Here's how the part is built. I have some questions about the finished solid (model axes, mm). Coordinates: 2 decimals unless noted, no trailing zeros. Write each loop counter-clockwise with the first axis right and the second up, starting at its lowest first coordinate (ties: lowest second). Pieces come first, ordered by that corner, then holes. Notation, with made-up numbers: (52.5, 71) -> (100.5, 71) arc R18 cw to (100.5, 86) -> close; hole circle Ø9 at (88, 40.25). An arc over 180 degrees is marked (long way). Use a Markdown table: item, result. Add a question column.
Item 1: Imagine slicing it at D-D, the plane x = 1.05. Count the separate pieces of the cut face and the enclosed holes in it, and give its area (3 significant figures).
Item 2: Imagine slicing it at B-B, the plane y = 10.3. Write out the boundary of the cut face in (x, z), and give its area (3 significant figures).
Item 3: Will this pin go through, and if not, where does the flat tip stop? pin 1 Ø0.7 at (x, y) = (1.5, 58) entering from -Z.
Item 4: Imagine slicing it at A-A, the plane z = -11. Write out the boundary of the cut face in (x, y).
Item 5: If I drill on line 1 along Z through (x, y) = (0.5, 19); line 2 along Z through (x, y) = (0.15, 40); line 3 along Y through (x, z) = (0.3, -95), over which ranges is the centre line in solid material (lowest first)? Write a range as from..to.
Item 6: Imagine slicing it at C-C, the plane y = 19.05. Write out the boundary of the cut face in (x, z).
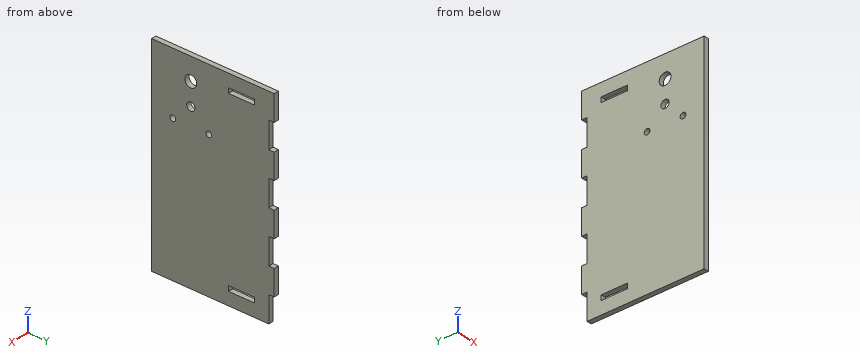
```python
from build123d import *

# Parameters (mm, degrees)
BOSS_EXTRUDE1_DEPTH = 2.3622
CUT_EXTRUDE1_REACH  = 4.362
SKETCH2_R           = 1.4
SKETCH2_R_2         = 2
SKETCH2_R_3         = 2.876999961
CUT_EXTRUDE2_DEPTH  = 3.3622
SKETCH4_W           = 2.4892
SKETCH4_H           = 12.7
CUT_EXTRUDE3_DEPTH  = 3.3622


with BuildPart() as part:
    # Sketch1 → Boss-Extrude1 (new body)
    with BuildSketch(Plane(origin=(0, 0, 0), x_dir=(0, 0, -1), z_dir=(1, 0, 0))):
        Polygon((0, 0), (0, 59.6392), (12.7, 59.6392), (12.7, 57.15), (25.4, 57.15), (25.4, 59.6392), (38.1, 59.6392), (38.1, 57.15), (50.8, 57.15), (50.8, 59.6392), (63.5, 59.6392), (63.5, 57.15), (76.2, 57.15), (76.2, 59.6392), (88.9, 59.6392), (88.9, 57.15), (101.6, 57.15), (101.6, 0), align=None)
    extrude(amount=BOSS_EXTRUDE1_DEPTH)

    # Sketch2 → Cut-Extrude1 (cut, up to next)
    with BuildSketch(Plane(origin=(2.3622, 0, 0), x_dir=(0, 0, -1), z_dir=(1, 0, 0)), mode=Mode.PRIVATE) as cut_extrude1_sk1:
        with Locations((30.59102, 10.3)):
            Circle(SKETCH2_R)
    cut_extrude1_tool1 = extrude(cut_extrude1_sk1.sketch, amount=-CUT_EXTRUDE1_REACH, mode=Mode.PRIVATE) & part.part
    add(cut_extrude1_tool1.solids().sort_by_distance((2.3622, 10.3, -30.59102))[0], mode=Mode.SUBTRACT)
    # Sketch2 → Cut-Extrude1 (cut, up to next)
    with BuildSketch(Plane(origin=(2.3622, 0, 0), x_dir=(0, 0, -1), z_dir=(1, 0, 0)), mode=Mode.PRIVATE) as cut_extrude1_sk2:
        with Locations((30.59102, 27.8)):
            Circle(SKETCH2_R)
    cut_extrude1_tool2 = extrude(cut_extrude1_sk2.sketch, amount=-CUT_EXTRUDE1_REACH, mode=Mode.PRIVATE) & part.part
    add(cut_extrude1_tool2.solids().sort_by_distance((2.3622, 27.8, -30.59102))[0], mode=Mode.SUBTRACT)
    # Sketch2 → Cut-Extrude1 (cut, up to next)
    with BuildSketch(Plane(origin=(2.3622, 0, 0), x_dir=(0, 0, -1), z_dir=(1, 0, 0)), mode=Mode.PRIVATE) as cut_extrude1_sk3:
        with Locations((22.0000034, 19.05)):
            Circle(SKETCH2_R_2)
    cut_extrude1_tool3 = extrude(cut_extrude1_sk3.sketch, amount=-CUT_EXTRUDE1_REACH, mode=Mode.PRIVATE) & part.part
    add(cut_extrude1_tool3.solids().sort_by_distance((2.3622, 19.05, -22.000003))[0], mode=Mode.SUBTRACT)
    # Sketch2 → Cut-Extrude1 (cut, up to next)
    with BuildSketch(Plane(origin=(2.3622, 0, 0), x_dir=(0, 0, -1), z_dir=(1, 0, 0)), mode=Mode.PRIVATE) as cut_extrude1_sk4:
        with Locations((11, 19.05)):
            Circle(SKETCH2_R_3)
    cut_extrude1_tool4 = extrude(cut_extrude1_sk4.sketch, amount=-CUT_EXTRUDE1_REACH, mode=Mode.PRIVATE) & part.part
    add(cut_extrude1_tool4.solids().sort_by_distance((2.3622, 19.05, -11))[0], mode=Mode.SUBTRACT)

    # Sketch3 → Cut-Extrude2 (cut, through all)
    with BuildSketch(Plane(origin=(2.3622, 0, 0), x_dir=(0, 0, -1), z_dir=(1, 0, 0))):
        Polygon((12.7, 57.15), (12.7, 59.6392), (12.573, 59.6392), (12.573, 57.023), (25.527, 57.023), (25.527, 59.6392), (25.4, 59.6392), (25.4, 57.15), align=None)
        Polygon((38.1, 59.6392), (37.973, 59.6392), (37.973, 57.023), (50.927, 57.023), (50.927, 59.6392), (50.8, 59.6392), (50.8, 57.15), (38.1, 57.15), align=None)
        Polygon((63.5, 59.6392), (63.373, 59.6392), (63.373, 57.023), (76.327, 57.023), (76.327, 59.6392), (76.2, 59.6392), (76.2, 57.15), (63.5, 57.15), align=None)
        Polygon((88.9, 59.6392), (88.773, 59.6392), (88.773, 57.023), (101.6, 57.023), (101.6, 57.15), (88.9, 57.15), align=None)
    extrude(amount=-CUT_EXTRUDE2_DEPTH, mode=Mode.SUBTRACT)

    # Sketch4 → Cut-Extrude3 (cut, through all)
    with BuildSketch(Plane(origin=(2.3622, 0, 0), x_dir=(0, 0, -1), z_dir=(1, 0, 0))):
        with Locations((7.5946, 43.7642)):
            Rectangle(SKETCH4_W, SKETCH4_H)
        with Locations((94.0054, 43.7642)):
            Rectangle(SKETCH4_W, SKETCH4_H)
    extrude(amount=-CUT_EXTRUDE3_DEPTH, mode=Mode.SUBTRACT)


solid = part.part
```
Ans:
| question | item | result |
|---|---|---|
| 1 | separate pieces | 1 |
| 1 | enclosed holes | 6 |
| 1 | area | 5,810 mm^2 |
| 2 | outline | (0, -101.6) -> (2.36, -101.6) -> (2.36, -31.99) -> (0, -31.99) -> close; (0, -29.19) -> (2.36, -29.19) -> (2.36, 0) -> (0, 0) -> close |
| 2 | area | 233 mm^2 |
| 3 | pin 1 | stops at z = -88.77 |
| 4 | outline | (0, 0) -> (2.36, 0) -> (2.36, 16.17) -> (0, 16.17) -> close; (0, 21.93) -> (2.36, 21.93) -> (2.36, 59.64) -> (0, 59.64) -> close |
| 5 | line 1 | z = -101.6..-24, -20..-13.88, -8.12..0 |
| 5 | line 2 | z = -101.6..-95.25, -92.76..-8.84, -6.35..0 |
| 5 | line 3 | y = 0..37.41, 50.11..57.02 |
| 6 | outline | (0, -101.6) -> (2.36, -101.6) -> (2.36, -24) -> (0, -24) -> close; (0, -20) -> (2.36, -20) -> (2.36, -13.88) -> (0, -13.88) -> close; (0, -8.12) -> (2.36, -8.12) -> (2.36, 0) -> (0, 0) -> close |
